Work out the finished part from the listing and answer in its coordinate system (mm). Round coordinates to 2 decimals unless told otherwise and drop trailing zeros. Order: outer loops, then holes, each group sorted by start corner. A loop starts at its lowest first (then second) coordinate and runs counter-clockwise, first axis right, second up. Notation, with made-up numbers: M 66,-15.75 L 98,-15.75 A5 cw 98,-8.75 Z; hole C -27.5,60 d2. An arc over 180 degrees is marked long. Answer as a JSON object with one key per item and string values. Group by question number.
from build123d import *

# Parameters (mm, degrees)
F0_R     = 2.7608867496
F0_W     = 19.05
F0_H     = 10.16
F0_R_2   = 1.5
F0_W_2   = 10.16
F0_H_2   = 19.05
F0_H_3   = 38.1
F1_DEPTH = 3.175


# Not quite as in the source:
# - a length typed as a fraction of an inch, garbled in the dataset ("3 / 203.2 mm" for 3/8 in), is restored


with BuildPart() as f1:
    # F0 (on Top) → F1 (new body)
    with BuildSketch(Plane.XY):
        with BuildLine():
            Line((100, 125), (-100, 125))
            ThreePointArc((-100, 125), (-117.6776695297, 117.6776695297), (-125, 100))
            Line((-125, 100), (-125, -100))
            ThreePointArc((-125, -100), (-117.6776695297, -117.6776695297), (-100, -125))
            Line((-100, -125), (100, -125))
            ThreePointArc((100, -125), (117.6776695297, -117.6776695297), (125, -100))
            Line((125, -100), (125, 100))
            ThreePointArc((125, 100), (117.6776695297, 117.6776695297), (100, 125))
        make_face()
        with Locations((-100, -100)):
            Circle(F0_R, mode=Mode.SUBTRACT)
        with Locations((-47.4411445916, -109.76)):
            Rectangle(F0_W, F0_H, mode=Mode.SUBTRACT)
        with Locations((-8.23, -113)):
            Circle(F0_R_2, mode=Mode.SUBTRACT)
        with Locations((-96.4635497928, -11.935)):
            Circle(F0_R_2, mode=Mode.SUBTRACT)
        with Locations((-66.9635497928, -11.935)):
            Circle(F0_R_2, mode=Mode.SUBTRACT)
        with Locations((8.23, -113)):
            Circle(F0_R_2, mode=Mode.SUBTRACT)
        with Locations((47.4411445916, -109.76)):
            Rectangle(F0_W, F0_H, mode=Mode.SUBTRACT)
        with Locations((100, -100)):
            Circle(F0_R, mode=Mode.SUBTRACT)
        with Locations((66.9635497928, -11.935)):
            Circle(F0_R_2, mode=Mode.SUBTRACT)
        with Locations((96.4635497928, -11.935)):
            Circle(F0_R_2, mode=Mode.SUBTRACT)
        with Locations((-109.76, 0)):
            Rectangle(F0_W_2, F0_H_2, mode=Mode.SUBTRACT)
        with Locations((-96.4635497928, 11.935)):
            Circle(F0_R_2, mode=Mode.SUBTRACT)
        with Locations((-66.9635497928, 11.935)):
            Circle(F0_R_2, mode=Mode.SUBTRACT)
        with Locations((-63.4532595247, 56.2142550719)):
            Rectangle(F0_W, F0_H_3, mode=Mode.SUBTRACT)
        with Locations((-100, 100)):
            Circle(F0_R, mode=Mode.SUBTRACT)
        with Locations((-47.4411445916, 109.76)):
            Rectangle(F0_W, F0_H, mode=Mode.SUBTRACT)
        with Locations((-8.23, 113)):
            Circle(F0_R_2, mode=Mode.SUBTRACT)
        with Locations((66.9635497928, 11.935)):
            Circle(F0_R_2, mode=Mode.SUBTRACT)
        with Locations((96.4635497928, 11.935)):
            Circle(F0_R_2, mode=Mode.SUBTRACT)
        with Locations((109.76, 0)):
            Rectangle(F0_W_2, F0_H_2, mode=Mode.SUBTRACT)
        with Locations((63.4532595247, 56.2142550719)):
            Rectangle(F0_W, F0_H_3, mode=Mode.SUBTRACT)
        with Locations((8.23, 113)):
            Circle(F0_R_2, mode=Mode.SUBTRACT)
        with Locations((47.4411445916, 109.76)):
            Rectangle(F0_W, F0_H, mode=Mode.SUBTRACT)
        with Locations((100, 100)):
            Circle(F0_R, mode=Mode.SUBTRACT)
    extrude(amount=F1_DEPTH)


solid = f1.part
Item 1: Each of these flat-tipped pins is pushed along its axis until it touches: pin 1 (1.6 mm diameter, centred on y = -110, z = 1, fed in from +X); pin 2 (1.8 mm diameter, centred on x = 96.46, y = 11.94, fed in from +Z). Where does it stop, or does it pass through?
Item 2: The mould has two halves that part along X. Classify faces 1 (the cylindrical face through (-117.482, 117.871, 1.565)), 2 (the cylindrical face through (117.871, 117.482, 1.565)), 3 (the flat face through (-2, 2, 0)), 4 (the cylindrical face through (99.641, 102.737, 1.565)): +X half, -X half, draft (parallel to the pull), parting line (faces both ways), or undercut.
Item 3: Consider L1, parallel to Y at x = 100, z = 1.65; L2, parallel to Y at x = -43, z = 1.75; L3, parallel to X at y = 57, z = 0.3. Determine where each line is inside the solid, lowest interval first.
Item 4: Find section C-C (z = 1). Give the number of separate pieces and of enclosed holes in the cut face, and give its area (3 significant figures).
Item 5: Find section A-A (y = 1). Give the vertices of the cut face in (x, z) (3 decimals), and give its area (3 significant figures).
Item 6: Find section B-B (y = 44). Give the vertices of the cut face in (x, z) (3 decimals).
Responses:
{
 "1": {"pin 1": "stops at x = 123.25", "pin 2": "passes through"},
 "2": {"face 1": "-X half", "face 2": "+X half", "face 3": "draft", "face 4": "undercut"},
 "3": {"L1": "y = -125 to -102.76, -97.24 to 97.24, 102.76 to 125", "L2": "y = -125 to -114.84, -104.68 to 104.68, 114.84 to 125", "L3": "x = -125 to -72.98, -53.93 to 53.93, 72.98 to 125"},
 "4": {"separate pieces": "1", "enclosed holes": "24", "area": "59,200 mm^2"},
 "5": {"outline": "M -125,0 L -114.84,0 L -114.84,3.175 L -125,3.175 Z; M -104.68,0 L 104.68,0 L 104.68,3.175 L -104.68,3.175 Z; M 114.84,0 L 125,0 L 125,3.175 L 114.84,3.175 Z", "area": "729 mm^2"},
 "6": {"outline": "M -125,0 L -72.978,0 L -72.978,3.175 L -125,3.175 Z; M -53.928,0 L 53.928,0 L 53.928,3.175 L -53.928,3.175 Z; M 72.978,0 L 125,0 L 125,3.175 L 72.978,3.175 Z"}
}
